Can you work these out from the drawing? Everything is in mm from the part's minimum corner. A direction names the side the tool comes from. Round coordinates to 2 decimals unless told otherwise and drop trailing zeros. Write each loop counter-clockwise with the first axis right and the second up, starting at its lowest first coordinate (ties: lowest second). Pieces come first, ordered by that corner, then holes. Notation, with made-up numbers: (8, -0.75) -> (38, -0.75) arc R30 cw to (38, 32.25) -> close; hole circle Ø10 at (11, 55). An arc over 180 degrees is marked (long way). Write item = value, one per line. Start each with the question number.
1) Imagine slicing it at A-A, the plane z = 121. Please give me the cut outline in (x, y), then the cut area to 3 significant figures.
2) Imagine slicing it at C-C, the plane y = 299. Please give me the cut outline in (x, z).
3) I'm going to push flat-ended pins straight in: pin 1 (7 mm diameter, centred on y = 325.5, z = 22, fed in from -X); pin 2 (1.5 mm diameter, centred on y = 244.5, z = 125, fed in from +X); pin 3 (12 mm diameter, centred on x = 323.5, y = 323, fed in from +Z). Where does each tip first touch, or does it pass through?
4) If I drill on line 1 (X direction, y = 287.5, z = 74); line 2 (Y direction, x = 121, z = 43.5); line 3 (Z direction, x = 244, y = 153), over which ranges is the centre line in solid material (lowest first)?
5) For the marked faces 4, 5 and 6, which set-ups out of +Z, -Z, +X, -X, +Y, -Y let a thin tool reach every point of the face, with its end or its side?
6) Thinking about a two-plate mould opening in Y: for the marked faces 1, 2 and 3, which applies, +Y half, -Y half, draft (parallel to the pull), parting line (faces both ways), or undercut?
7) Imagine slicing it at B-B, the plane x = 248.5. Please give me the cut outline in (y, z).
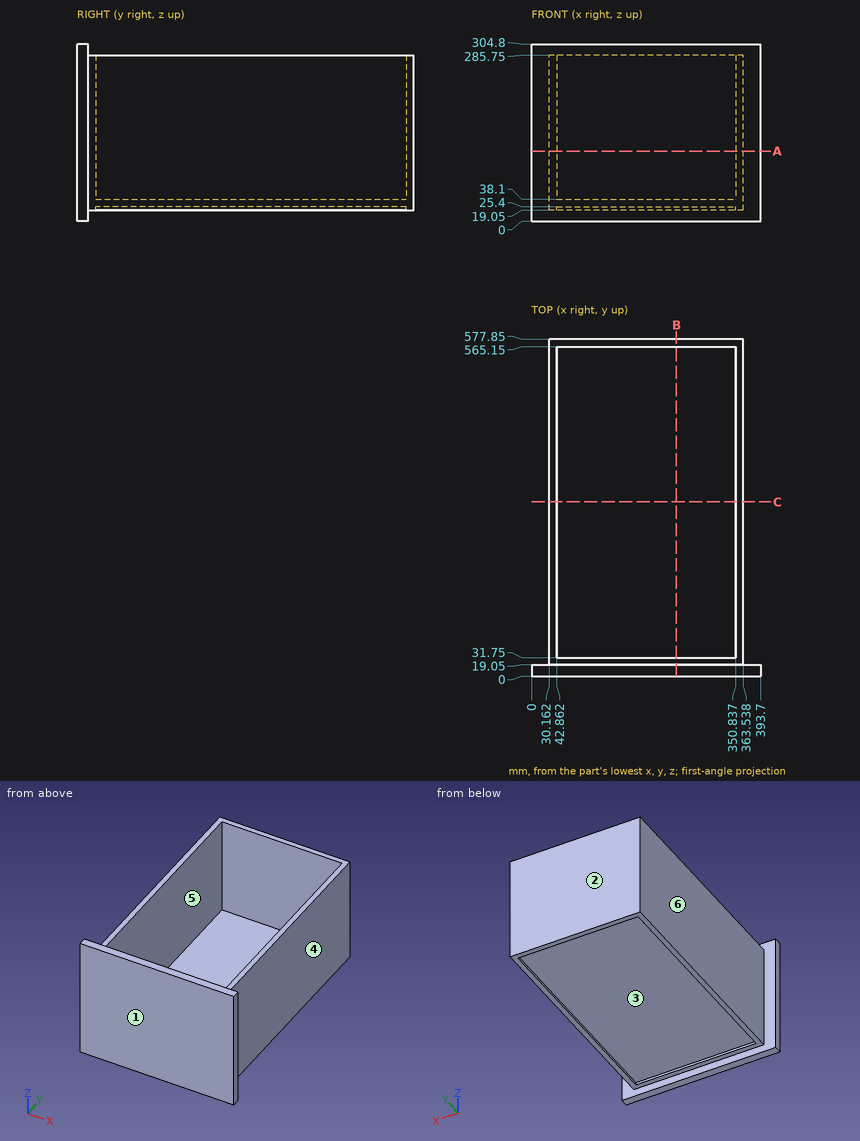
Reported:
q1.outline = (0, 0) -> (393.7, 0) -> (393.7, 19.05) -> (363.54, 19.05) -> (363.54, 577.85) -> (30.16, 577.85) -> (30.16, 19.05) -> (0, 19.05) -> close; hole (42.86, 31.75) -> (350.84, 31.75) -> (350.84, 565.15) -> (42.86, 565.15) -> close
q1.area = 29,500 mm²
q2.outline = (30.16, 19.05) -> (42.86, 19.05) -> (42.86, 25.4) -> (350.84, 25.4) -> (350.84, 19.05) -> (363.54, 19.05) -> (363.54, 285.75) -> (350.84, 285.75) -> (350.84, 38.1) -> (42.86, 38.1) -> (42.86, 285.75) -> (30.16, 285.75) -> close
q3.pin_1 = 30.16
q3.pin_2 = 363.54
q3.pin_3 = 38.1
q4.line_1 = 30.16 to 42.86, 350.84 to 363.54
q4.line_2 = 0 to 31.75, 565.15 to 577.85
q4.line_3 = 25.4 to 38.1
q5.face_4 = +Z, -Z, +X, +Y
q5.face_5 = +Z
q5.face_6 = +Z, -Z, -X, +Y
q6.face_1 = -Y half
q6.face_2 = +Y half
q6.face_3 = undercut
q7.outline = (0, 0) -> (19.05, 0) -> (19.05, 19.05) -> (31.75, 19.05) -> (31.75, 25.4) -> (565.15, 25.4) -> (565.15, 19.05) -> (577.85, 19.05) -> (577.85, 285.75) -> (565.15, 285.75) -> (565.15, 38.1) -> (31.75, 38.1) -> (31.75, 285.75) -> (19.05, 285.75) -> (19.05, 304.8) -> (0, 304.8) -> close
